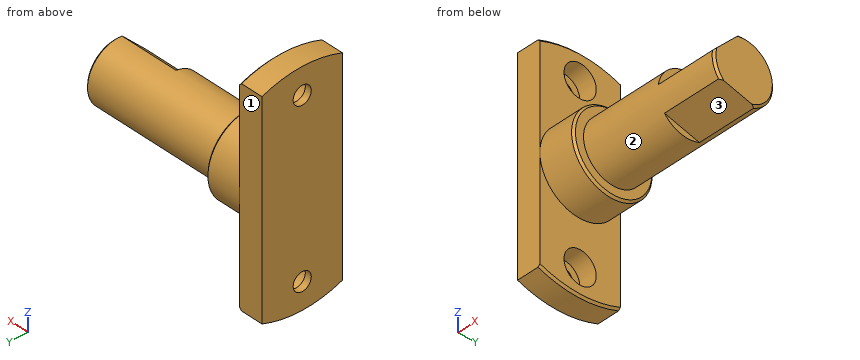
from build123d import *

# Parameters (mm, degrees)
CHANFREIN1_SIZE                                    = 0.5
CHAMBRAGE_POUR_VIS_T_TE_HEXAGONALE_M41_D           = 4.5
CHAMBRAGE_POUR_VIS_T_TE_HEXAGONALE_M41_CBORE_D     = 8
CHAMBRAGE_POUR_VIS_T_TE_HEXAGONALE_M41_CBORE_DEPTH = 4.4
ENL_V_MAT_EXTRU_1_DEPTH                            = 15
ENL_V_MAT_EXTRU_2_DEPTH                            = 64.344297297
CHANFREIN3_SIZE                                    = 0.5


with BuildPart() as part:
    # Esquisse1 → Révolution1 (revolve)
    with BuildSketch(Plane.XY):
        Polygon((15, 7.5), (50, 7.5), (50, 0), (0, 0), (0, 27.5), (6, 27.5), (6, 10), (15, 10), align=None)
    revolve(axis=Axis((50, 0, 0), (-1, 0, 0)))

    # Chanfrein1
    chanfrein1_edges = [part.edges().sort_by_distance(p)[0] for p in [
        (6, -27.5, 0),
        (15, -10, 0),
    ]]
    chamfer(chanfrein1_edges, length=CHANFREIN1_SIZE)

    # Chambrage pour vis à tête hexagonale M41 (through all)
    with Locations(Plane(origin=(6, 0, 0), x_dir=(0, 0, -1), z_dir=(1, 0, 0))):
        with Locations((-21, 0), (21, 0)):
            CounterBoreHole(CHAMBRAGE_POUR_VIS_T_TE_HEXAGONALE_M41_D / 2, CHAMBRAGE_POUR_VIS_T_TE_HEXAGONALE_M41_CBORE_D / 2, CHAMBRAGE_POUR_VIS_T_TE_HEXAGONALE_M41_CBORE_DEPTH)

    # Esquisse8 → Enlèv. mat.-Extru.1 (cut)
    with BuildSketch(Plane(origin=(50, 0, 0), x_dir=(0, 0, -1), z_dir=(1, 0, 0))):
        with BuildLine():
            Line((-1.060660172, -7.424621202), (-7.424621202, -1.060660172))
            ThreePointArc((-7.424621202, -1.060660172), (-5.303300859, -5.303300859), (-1.060660172, -7.424621202))
        make_face()
        with BuildLine():
            Line((4.630869255, -5.899580489), (6.960240661, 2.793751948))
            ThreePointArc((6.960240661, 2.793751948), (7.244443697, -1.941142838), (4.630869255, -5.899580489))
        make_face()
    extrude(amount=-ENL_V_MAT_EXTRU_1_DEPTH, mode=Mode.SUBTRACT)

    # Esquisse11 → Enlèv. mat.-Extru.2 (cut, through all)
    with BuildSketch(Plane.ZY):
        with BuildLine():
            Line((25.617376915, -10), (-25.617376915, -10))
            ThreePointArc((-25.617376915, -10), (0, -27.5), (25.617376915, -10))
        make_face()
        with BuildLine():
            Line((25.617376915, 10), (-25.617376915, 10))
            ThreePointArc((-25.617376915, 10), (0, 27.5), (25.617376915, 10))
        make_face()
    extrude(amount=-ENL_V_MAT_EXTRU_2_DEPTH, mode=Mode.SUBTRACT)

    # Chanfrein3
    chanfrein3_edges = [part.edges().sort_by_distance(p)[0] for p in [
        (50, -7.244443697, -1.941142838),
        (50, 4.91401306, 5.665904662),
    ]]
    chamfer(chanfrein3_edges, length=CHANFREIN3_SIZE)


solid = part.part
The model under review builds one solid part; all positions refer to its coordinate system, in mm. Face numbers are marked on the shaded views. A direction names the side the tool comes from. Give positions to 0.01 mm unless a question says otherwise; leave off trailing zeros. Loops run counter-clockwise (first coordinate to the right, second up) from the corner with the lowest first, then second, coordinate; pieces in that order, holes last. Notation, with made-up numbers: (6, 72) -> (38, 72) arc R15 ccw to (38, 101) -> close; hole circle Ø1 at (-37, 15). An arc over 180 degrees is marked (long way). Put each result on its own line as item: value. Start each with the question number.
1. We need section C-C on x = 9. State the section outline as (y, z) points, then the cut area to 3 significant figures.
2. We need section D-D on y = 0. State how many separate pieces and enclosed holes the cut face has, then the cut area to 3 significant figures.
3. For the marked faces 1, 2 and 3, list the 3-axis set-ups (+Z, -Z, +X, -X, +Y, -Y) from which the entire face can be reached by the end or side of a thin tool; tool diameter is ignored.
4. Wall thickness on probe 1 along Y at (x, z) = (3, -21); probe 2 along Y at (x, z) = (1, -21); probe 3 along Z at (x, y) = (25, -1): over which ranges is each line inside the solid? List them lowest first.
5. We need section B-B on z = -24. State the section outline as (x, y) points.
6. Clearance check with flat-ended pins moving along their axes: P1, Ø5, axis at x = 23, z = 1, coming from the +Y side; P2, Ø3.5, axis at y = 0, z = -21, coming from the -X side; P3, Ø6.5, axis at y = -1.5, z = -21.5, coming from the +X side; P4, Ø12, axis at x = 30.5, y = -7, coming from the +Z side. State where each tip first meets the part, or that it passes through.
7. We need section A-A on z = 21. State the section outline as (x, y) points.
Determined:
1. outline: circle Ø20 at (0, 0)
1. area: 314 mm^2
2. separate pieces: 3
2. enclosed holes: 0
2. area: 930 mm^2
3. face 1: +Z, -Z, +X, -X, +Y
3. face 2: +X
3. face 3: -Z, +X, -Y
4. probe 1: -10 to -4, 4 to 10
4. probe 2: -10 to -2.25, 2.25 to 10
4. probe 3: -7.43 to 7.43
5. outline: (0, -10) -> (6, -10) -> (6, -2.65) -> (1.6, -2.65) -> (1.6, 2.65) -> (6, 2.65) -> (6, 10) -> (0, 10) -> close
6. P1: y = 7.5
6. P2: through
6. P3: x = 6
6. P4: z = 7.43
7. outline: (0, -10) -> (6, -10) -> (6, -4) -> (1.6, -4) -> (1.6, -2.25) -> (0, -2.25) -> close; (0, 2.25) -> (1.6, 2.25) -> (1.6, 4) -> (6, 4) -> (6, 10) -> (0, 10) -> close
